from build123d import *

# Parameters (mm, degrees)
SKETCH1_W             = 16
SKETCH1_H             = 12
BOSS_EXTRUDE1_DEPTH   = 5.5
SKETCH2_W             = 0.6
SKETCH2_H             = 12
SKETCH2_W_2           = 1.5
BOSS_EXTRUDE2_DEPTH   = 5
FILLET1_R             = 0.5
M3_TAPPED_HOLE1_D     = 2.5
M3_TAPPED_HOLE1_DEPTH = 10
M3_TAPPED_HOLE1_TIP   = 0.751075774


with BuildPart() as part:
    # Sketch1 → Boss-Extrude1 (new body)
    with BuildSketch(Plane(origin=(0, 0, 0), x_dir=(1, 0, 0), z_dir=(0, 1, 0))):
        Rectangle(SKETCH1_W, SKETCH1_H)
    extrude(amount=BOSS_EXTRUDE1_DEPTH)

    # Sketch2 → Boss-Extrude2 (add)
    with BuildSketch(Plane(origin=(0, 5.5, 0), x_dir=(1, 0, 0), z_dir=(0, 1, 0))):
        with Locations((-7.7, 0)):
            Rectangle(SKETCH2_W, SKETCH2_H)
        with Locations((7.7, 0)):
            Rectangle(SKETCH2_W, SKETCH2_H)
        Rectangle(SKETCH2_W_2, SKETCH2_H)
    extrude(amount=BOSS_EXTRUDE2_DEPTH)

    # Fillet1
    fillet1_edges = [part.edges().sort_by_distance(p)[0] for p in [
        (-7.7, 10.5, 6),
        (-7.7, 10.5, -6),
        (7.7, 10.5, -6),
        (7.7, 10.5, 6),
        (0, 10.5, 6),
        (0, 10.5, -6),
    ]]
    fillet(fillet1_edges, radius=FILLET1_R)

    # M3 Tapped Hole1
    with Locations(Plane(origin=(0, 5.5, 0), x_dir=(1, 0, 0), z_dir=(0, 1, 0))):
        with Locations((-4.075, 0), (4.075, 0)):
            Hole(M3_TAPPED_HOLE1_D / 2, depth=M3_TAPPED_HOLE1_DEPTH)
            with Locations((0, 0, -(M3_TAPPED_HOLE1_DEPTH + M3_TAPPED_HOLE1_TIP / 2))):  # 118° drill point
                Cone(0, M3_TAPPED_HOLE1_D / 2, M3_TAPPED_HOLE1_TIP, mode=Mode.SUBTRACT)


solid = part.part
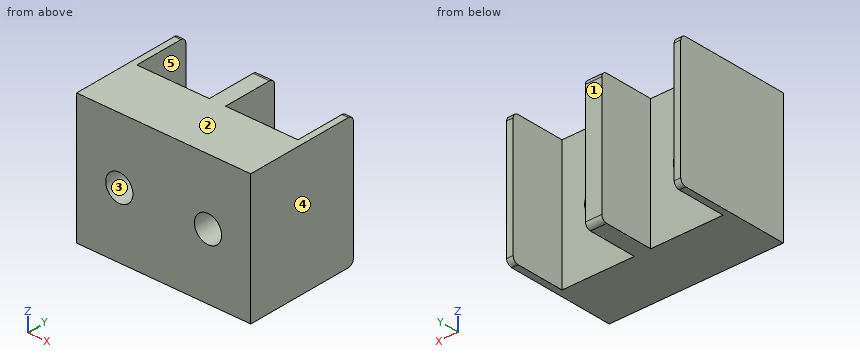
Geometry: final body of the model. Coordinates: model frame, mm. Face numbers are marked on the shaded views. A direction names the side the tool comes from. Give positions to 0.01 mm unless a question says otherwise; leave off trailing zeros. Order: outer loops, then holes, each group sorted by start corner. A loop starts at its lowest first (then second) coordinate and runs counter-clockwise, first axis right, second up. Notation, with made-up numbers: (-20.75, 87.25) -> (-0.75, 87.25) arc R25 cw to (-0.75, 105.25) -> close; hole circle Ø8 at (38, 87). An arc over 180 degrees is marked (long way). Answer as a JSON object with one key per item and string values.
Q1. Section C-C (x = -3.5). Output: boundary loops of the cut face in (y, z), plus the area to 3 significant figures.
Entries:
{"outline": "(0, -6) -> (5.5, -6) -> (5.5, -1.11) -> (0, -1.11) -> close; (0, 1.11) -> (5.5, 1.11) -> (5.5, 6) -> (0, 6) -> close", "area": "53.8 mm^2"}
Q2. Section D-D (z = -4). Output: boundary loops of the cut face in (x, y).
Entries:
{"outline": "(-8, 0) -> (8, 0) -> (8, 10.5) -> (7.4, 10.5) -> (7.4, 5.5) -> (0.75, 5.5) -> (0.75, 10.5) -> (-0.75, 10.5) -> (-0.75, 5.5) -> (-7.4, 5.5) -> (-7.4, 10.5) -> (-8, 10.5) -> close"}
Q3. Section B-B (z = 0). Output: boundary loops of the cut face in (x, y) (3 decimals).
Entries:
{"outline": "(-8, 0) -> (-5.325, 0) -> (-5.325, 5.5) -> (-7.4, 5.5) -> (-7.4, 10.5) -> (-8, 10.5) -> close; (-2.825, 0) -> (2.825, 0) -> (2.825, 5.5) -> (0.75, 5.5) -> (0.75, 10.5) -> (-0.75, 10.5) -> (-0.75, 5.5) -> (-2.825, 5.5) -> close; (5.325, 0) -> (8, 0) -> (8, 10.5) -> (7.4, 10.5) -> (7.4, 5.5) -> (5.325, 5.5) -> close"}
Q4. First-contact query: pin 1 (3 mm diameter, centred on x = -4.5, y = 8.5, fed in from +Z); pin 2 (2 mm diameter, centred on x = 2.5, z = 2.5, fed in from +Y). Flat tips, straight axial feed; report the tip coordinate or a pass-through.
Entries:
{"pin 1": "passes through", "pin 2": "stops at y = 5.5"}
Q5. Section A-A (y = 7.75). Output: boundary loops of the cut face in (x, z), plus the area to 3 significant figures.
Entries:
{"outline": "(-8, -6) -> (-7.4, -6) -> (-7.4, 6) -> (-8, 6) -> close; (-0.75, -6) -> (0.75, -6) -> (0.75, 6) -> (-0.75, 6) -> close; (7.4, -6) -> (8, -6) -> (8, 6) -> (7.4, 6) -> close", "area": "32.4 mm^2"}
Q6. Material intervals for probe 1 along X at (y, z) = (7.5, 5); probe 2 along Y at (x, z) = (6.5, 3.5); probe 3 along Z at (x, y) = (5, 4.75), sorted ascending.
Entries:
{"probe 1": "x = -8 to -7.4, -0.75 to 0.75, 7.4 to 8", "probe 2": "y = 0 to 5.5", "probe 3": "z = -6 to -0.84, 0.84 to 6"}
Q7. Access query for the marked faces 4 and 5. Directions: +Z, -Z, +X, -X, +Y, -Y. A direction counts if a zero-diameter tool reaches every point of the face in a straight line with its end or side. Return the directions, or none.
Entries:
{"face 4": "+Z, -Z, +X, +Y, -Y", "face 5": "+Z, -Z, +Y"}
Q8. Draft query along Z for the marked faces 1, 2 and 3. Return one class per face: released by +Z, released by -Z, zero draft, split by the parting line, or undercut.
Entries:
{"face 1": "zero draft", "face 2": "released by +Z", "face 3": "undercut"}
